```python
from build123d import *

# Parameters (mm, degrees)
F1_DEPTH = 44
F4_T     = -1.2
F3_R     = 17
F5_DEPTH = 25
F6_W     = 3.4
F6_H     = 40
F7_DEPTH = 50


with BuildPart() as f1:
    # F0 (on Front) → F1 (new body)
    with BuildSketch(Plane.XZ):
        Polygon((-3, 38.157568), (-15, 0), (15, 0), (3, 38.157568), align=None)
    extrude(amount=F1_DEPTH)

    # F4
    f4_openings = [f1.faces().sort_by_distance(p)[0] for p in [
        (0, -22, 0),
    ]]
    offset(amount=F4_T, openings=f4_openings)

    # F3 (on offset) → F5 (cut, symmetric)
    with BuildSketch(Plane.XZ.offset(25)):
        with Locations((0, -9)):
            Circle(F3_R)
    extrude(amount=F5_DEPTH, both=True, mode=Mode.SUBTRACT)

    # F6 (on Top) → F7 (cut)
    with BuildSketch(Plane.XY):
        with Locations((0.101443, -22.319711)):
            Rectangle(F6_W, F6_H)
    extrude(amount=F7_DEPTH, mode=Mode.SUBTRACT)


solid = f1.part
```
Here's how the part is built. I have some questions about the finished solid (model axes, mm). A direction names the side the tool comes from. Round coordinates to 2 decimals unless told otherwise and drop trailing zeros. Order: outer loops, then holes, each group sorted by start corner. A loop starts at its lowest first (then second) coordinate and runs counter-clockwise, first axis right, second up. Notation, with made-up numbers: M -29.75,4 L 17.25,4 A17 ccw 17.25,13 Z; hole C 67,8 d2. An arc over 180 degrees is marked long. One line per question, with ' | ' between items.
1) I want a section at A-A, the plane y = -30.5. Write out the boundary of the cut face in (x, z), then the cut area to 3 significant figures.
Working result:
outline: M -15,0 L -14.42,0 A17 cw -13.21,1.71 L -2.12,36.96 L -1.6,36.96 L -1.6,38.16 L -3,38.16 Z; M 1.8,36.96 L 2.12,36.96 L 13.21,1.71 A17 cw 14.42,0 L 15,0 L 3,38.16 L 1.8,38.16 Z | area: 95.3 mm²
2) I want a section at C-C, the plane x = -0.25. Write out the boundary of the cut face in (y, z).
Working result:
outline: M -44,8 L -42.8,8 L -42.8,36.96 L -42.32,36.96 L -42.32,38.16 L -44,38.16 Z; M -2.32,36.96 L -1.2,36.96 L -1.2,8 L 0,8 L 0,38.16 L -2.32,38.16 Z
3) I need wall thicknesses on line 1 along Y through (x, z) = (-0.25, 34.5); line 2 along X through (y, z) = (-32, 11.5); line 3 along X through (y, z) = (-7, 3.5). Which ranges of each line are inside material? Lowest first, please.
Working result:
line 1: -44 to -42.8, -1.2 to 0 | line 2: -11.38 to -10.13, 10.13 to 11.38 | line 3: -13.9 to -12.64, 12.64 to 13.9
4) For pin 1 Ø10 at (y, z) = (-5, 21.5) entering from -X; pin 2 Ø1 at (x, z) = (0, 20) entering from +Y; pin 3 Ø10 at (x, y) = (8.5, -27.5) entering from -Z; pin 4 Ø1.5 at (y, z) = (-29.5, 19) entering from +X, each with a flat end and sliding along its axis, tell me the tip position at first contact or that it passes through.
Working result:
pin 1: x = -9.81 | pin 2: y = 0 | pin 3: z = 1.33 | pin 4: x = 9.26
5) I want a section at B-B, the plane z = 27. Write out the boundary of the cut face in (x, y), then the cut area to 3 significant figures.
Working result:
outline: M -6.51,-44 L 6.51,-44 L 6.51,0 L -6.51,0 Z; hole M -5.25,-42.8 L 5.25,-42.8 L 5.25,-1.2 L -5.25,-1.2 Z | area: 136 mm²
6) For faces 4 (the face through (0, -42.8, 16)), 5 (the face through (-1.599, -23, 38)), 6 (the face through (0, -44, 19)), which set-ups out of +Z, -Z, +X, -X, +Y, -Y let a thin tool reach every point of the face, with its end or its side?
Working result:
face 4: -Z | face 5: +Z, -Z | face 6: +Z, -Z, +X, -X, -Y
7) If we mould it in two halves opening along X, with no side actions, what happens to faces 1 (the face through (7.74, -21.71, 19.08)), 2 (the face through (0, 0, 19)), 3 (the face through (-8.916, -21.692, 19.346))? For each: +X half, -X half, draft (parallel to the pull), parting line (faces both ways), or undercut.
Working result:
face 1: undercut | face 2: draft | face 3: -X half
8) I want a section at D-D, the plane z = 3. Write out the boundary of the cut face in (x, y), then the cut area to 3 significant figures.
Working result:
outline: M -14.06,-44 L -12.04,-44 L -12.04,-42.8 L -12.8,-42.8 L -12.8,-1.2 L -12.04,-1.2 L -12.04,0 L -14.06,0 Z; M 12.04,-44 L 14.06,-44 L 14.06,0 L 12.04,0 L 12.04,-1.2 L 12.8,-1.2 L 12.8,-42.8 L 12.04,-42.8 Z | area: 114 mm²
